from build123d import *

# Parameters (mm, degrees)
F1_DEPTH = 127
F2_W     = 19.05
F2_H     = 107.95
F3_DEPTH = 107.95
F4_R     = 19.05
F6_DEPTH = 25.4


with BuildPart() as f1:
    # F0 (on Front) → F1 (new body)
    with BuildSketch(Plane.XZ):
        Polygon((0, 127), (0, 0), (127, 0), (127, 19.05), (19.05, 19.05), (19.05, 127), align=None)
    extrude(amount=F1_DEPTH)

    # F2 (on face) → F3 (join, through all)
    with BuildSketch(Plane.YZ.offset(19.05)):
        with Locations((-63.5, 73.025)):
            Rectangle(F2_W, F2_H)
    extrude(amount=F3_DEPTH)

    # F4
    f4_edges = [f1.edges().sort_by_distance(p)[0] for p in [
        (127, -63.5, 127),
    ]]
    fillet(f4_edges, radius=F4_R)

    # F5 (on face) → F6 (cut)
    with BuildSketch(Plane.XZ.offset(73.025)):
        with BuildLine():
            ThreePointArc((77.897624, 89.627843), (81.555843, 77.027996), (94.407624, 74.387843))
            ThreePointArc((94.407624, 74.387843), (116.012004, 62.505843), (102.442376, 83.092157))
            ThreePointArc((102.442376, 83.092157), (98.784157, 95.692004), (85.932376, 98.332157))
            ThreePointArc((85.932376, 98.332157), (64.327996, 110.214157), (77.897624, 89.627843))
        make_face()
    extrude(amount=-F6_DEPTH, mode=Mode.SUBTRACT)


solid = f1.part
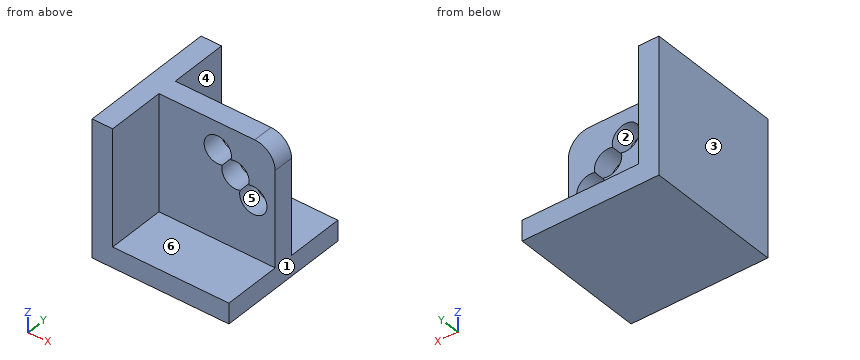
Can you work these out from the model? Positions are in its coordinate system, mm. Face numbers are marked on the shaded views. A direction names the side the tool comes from. Round coordinates to 2 decimals unless told otherwise and drop trailing zeros. Order: outer loops, then holes, each group sorted by start corner. A loop starts at its lowest first (then second) coordinate and runs counter-clockwise, first axis right, second up. Notation, with made-up numbers: M 32.25,0.5 L 49.25,0.5 A31 ccw 49.25,39.5 Z; hole C 1.5,51.5 d8. An arc over 180 degrees is marked long. Use a Markdown table: item, result.
1) Imagine slicing it at D-D (z = 49.5). List the corners of the cut face in (x, y) for me (3 decimals).
Geometry says:
| item | result |
|---|---|
| outline | M 0,-127 L 19.05,-127 L 19.05,-73.025 L 127,-73.025 L 127,-53.975 L 19.05,-53.975 L 19.05,0 L 0,0 Z |
2) I'm going to push flat-ended pins straight in: P1, Ø3, axis at x = 103, z = 25, coming from the -Y side (3 decimals); P2, Ø3, axis at y = -24.5, z = 31, coming from the +X side; P3, Ø10, axis at x = 42, z = 111.5, coming from the +Y side (3 decimals). Where does each tip first touch, or does it pass through?
Geometry says:
| item | result |
|---|---|
| P1 | stops at y = -73.025 |
| P2 | stops at x = 19.05 |
| P3 | stops at y = -53.975 |
3) On a 3-axis mill with a long thin cutter (end or side, diameter ignored), from which of +Z, -Z, +X, -X, +Y, -Y can I reach the whole of each face in a straight line? I mean the marked faces 4, 5 and 6. Say none if no direction works.
Geometry says:
| item | result |
|---|---|
| face 4 | +Z, +X, +Y |
| face 5 | +Y, -Y |
| face 6 | +Z, +X, -Y |
4) Imagine slicing it at C-C (y = -58.5). List the corners of the cut face in (x, z) for me, then the cut area to 3 significant figures.
Geometry says:
| item | result |
|---|---|
| outline | M 0,0 L 127,0 L 127,107.95 A19.05 ccw 107.95,127 L 0,127 Z; hole M 77.9,89.63 A12.7 ccw 94.41,74.39 A12.7 ccw long 102.44,83.09 A12.7 ccw 85.93,98.33 A12.7 ccw long Z |
| area | 14,600 mm² |
5) If I drill on line 1 along Z through (x, y) = (106.68, -65.75); line 2 along X through (y, z) = (-63.5, 71.12); line 3 along Z through (x, y) = (111, -80), over which ranges is the centre line in solid material (lowest first)?
Geometry says:
| item | result |
|---|---|
| line 1 | z = 0 to 58.42, 83.82 to 127 |
| line 2 | x = 0 to 93.98, 119.38 to 127 |
| line 3 | z = 0 to 19.05 |
6) Imagine slicing it at B-B (z = 71.12). List the corners of the cut face in (x, y) for me (3 decimals), then the cut area to 3 significant figures.
Geometry says:
| item | result |
|---|---|
| outline | M 0,-127 L 19.05,-127 L 19.05,-73.025 L 93.98,-73.025 L 93.98,-53.975 L 19.05,-53.975 L 19.05,0 L 0,0 Z; M 119.38,-73.025 L 127,-73.025 L 127,-53.975 L 119.38,-53.975 Z |
| area | 3,990 mm² |
7) If we mould it in two halves opening along X, with no side actions, what happens to the marked faces 1, 2 and 3? For each: +X half, -X half, draft (parallel to the pull), parting line (faces both ways), or undercut.
Geometry says:
| item | result |
|---|---|
| face 1 | +X half |
| face 2 | undercut |
| face 3 | -X half |
8) Imagine slicing it at A-A (x = 73.66). List the corners of the cut face in (y, z) for me (3 decimals), then the cut area to 3 significant figures.
Geometry says:
| item | result |
|---|---|
| outline | M -127,0 L 0,0 L 0,19.05 L -53.975,19.05 L -53.975,88.9 L -73.025,88.9 L -73.025,19.05 L -127,19.05 Z; M -73.025,114.3 L -53.975,114.3 L -53.975,127 L -73.025,127 Z |
| area | 3,990 mm² |
